```python
from build123d import *

# Parameters (mm, degrees)
SKETCH1_R           = 4
BOSS_EXTRUDE1_DEPTH = 13
SKETCH2_R           = 0.133652149
SKETCH2_R_2         = 0.154729583
BOSS_EXTRUDE2_DEPTH = 6


with BuildPart() as part:
    # Sketch1 → Boss-Extrude1 (new body)
    with BuildSketch(Plane(origin=(0, 0, 0), x_dir=(1, 0, 0), z_dir=(0, 1, 0))):
        with Locations(Location((0, 0, 0), (0, 0, 90))):
            Circle(SKETCH1_R)
    extrude(amount=BOSS_EXTRUDE1_DEPTH)

    # Sketch2 → Boss-Extrude2 (add)
    with BuildSketch(Plane.XZ):
        with Locations(Location((-2.639629951, 0, 0), (0, 0, 90))):
            Circle(SKETCH2_R)
        with Locations(Location((2.561666197, 0, 0), (0, 0, 90))):
            Circle(SKETCH2_R_2)
    extrude(amount=BOSS_EXTRUDE2_DEPTH)


solid = part.part
```
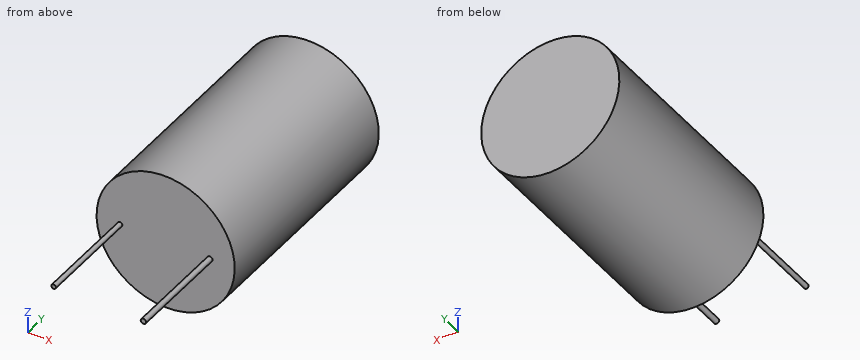
Input: part model. Units: mm. Frame: model coordinates. Coordinates: 2 decimals unless noted, no trailing zeros. Order: outer loops, then holes, each group sorted by start corner. A loop starts at its lowest first (then second) coordinate and runs counter-clockwise, first axis right, second up. Notation, with made-up numbers: (17, 79.25) - (63, 79.25) arc R20 cw to (63, 97.25) - close; hole circle Ø7 at (16, 53.5). An arc over 180 degrees is marked (long way). Put each result on its own line as item: value.
1. Cut plane A-A on x = 0. Return the cut outline in (y, z).
Report:
outline: (0, -4) - (13, -4) - (13, 4) - (0, 4) - close
2. Line query: line 1 along Y through (x, z) = (1, -3.5); line 2 along X through (y, z) = (3.25, -0.5); line 3 along Z through (x, y) = (-3, 5.5). Output: solid intervals per line, ascending.
Report:
line 1: y = 0 to 13
line 2: x = -3.97 to 3.97
line 3: z = -2.65 to 2.65
3. Contact query for flat-ended pins moving along their axis: pin 1 Ø2 at (y, z) = (9.5, -2.5) entering from +X; pin 2 Ø4 at (x, z) = (-0.5, -0.5) entering from -Y; pin 3 Ø3 at (x, y) = (-2, 7) entering from -Z. Output: stop coordinate, or through.
Report:
pin 1: stops at x = 3.71
pin 2: stops at y = 0
pin 3: stops at z = -3.97
4. Cut plane B-B on y = 2.25. Return the cut outline in (x, z).
Report:
outline: circle Ø8 at (0, 0)
5. Cut plane C-C on z = 0.5. Return the cut outline in (x, y), then the cut area to 3 significant figures.
Report:
outline: (-3.97, 0) - (3.97, 0) - (3.97, 13) - (-3.97, 13) - close
area: 103 mm2
